from build123d import *

# Parameters (mm, degrees)
SKETCH_1_W          = 11
SKETCH_1_H          = 36
EXTRUDE_1_DEPTH     = 18
SKETCH_2_R          = 7.5
EXTRUDE_2_DEPTH     = 20
FILLET_3_R          = 4
SKETCH_3_R          = 1.5
CUT_EXTRUDE_1_DEPTH = 45.944410108


with BuildPart() as part:
    # 草图1 → 凸台-拉伸1 (new, symmetric)
    with BuildSketch(Plane(origin=(0, 0, 0), x_dir=(0, 0, -1), z_dir=(1, 0, 0))):
        Rectangle(SKETCH_1_W, SKETCH_1_H)
    extrude(amount=EXTRUDE_1_DEPTH, both=True)

    # 草图2 → 凸台-拉伸2 (add)
    with BuildSketch(Plane.XY):
        with Locations(Location((0, 0, 0), (0, 0, 180))):
            Circle(SKETCH_2_R)
    extrude(amount=EXTRUDE_2_DEPTH)

    # 圆角3
    fillet_3_edges = [part.edges().sort_by_distance(p)[0] for p in [
        (7.5, 0, 20),
    ]]
    fillet(fillet_3_edges, radius=FILLET_3_R)

    # 草图3 → 切除-拉伸1 (cut, through all)
    with BuildSketch(Plane.ZY.offset(18)):
        Circle(SKETCH_3_R)
    extrude(amount=-CUT_EXTRUDE_1_DEPTH, mode=Mode.SUBTRACT)


solid = part.part
Model file for the job. Use its own axes, mm. Give positions to 0.01 mm unless a question says otherwise; leave off trailing zeros. Write each loop counter-clockwise with the first axis right and the second up, starting at its lowest first coordinate (ties: lowest second). Pieces come first, ordered by that corner, then holes. Notation, with made-up numbers: (69.5, 68.5) -> (106.5, 68.5) arc R11 ccw to (106.5, 82.5) -> close; hole circle Ø7 at (23, -34). An arc over 180 degrees is marked (long way). Write item = value, one per line.
(1) Slice it at D-D, the plane y = -8. Give the cut face in (x, z).
Determined:
outline = (-18, -5.5) -> (18, -5.5) -> (18, 5.5) -> (-18, 5.5) -> close
(2) Probe line 1 along Y through (x, z) = (1.5, 0); line 2 along Z through (x, y) = (11.5, -4.5); line 3 along Y through (x, z) = (0.5, 12.5). List the from-to ranges inside material, lowest first.
Determined:
line_1 = -18 to -1.5, 1.5 to 18
line_2 = -5.5 to 5.5
line_3 = -7.48 to 7.48
(3) Flat gauge pins, fed straight in: P1, Ø2, axis at x = 10, z = 14, coming from the +Y side; P2, Ø1.5, axis at x = -7.5, z = 13.5, coming from the -Y side; P3, Ø8, axis at x = 3, z = 11.5, coming from the -Y side; P4, Ø1, axis at x = 11, y = 6, coming from the +Z side. Where does each tip first touch, or does it go through?
Determined:
P1 = through
P2 = -3.27
P3 = -7.5
P4 = 5.5
(4) Mould opens along Z. For faces 1 (the face through (0, -8, 5.5)), 2 (the face through (-4.032, -6.324, 10.676)), 3 (the face through (-0.25, 0.07, -1.5)) say: released by +Z, released by -Z, zero draft, split by the parting line, or undercut.
Determined:
face_1 = released by +Z
face_2 = zero draft
face_3 = undercut
(5) Slice it at C-C, the plane z = 10.75. Give the cut face in (x, y), then the cut area to 3 significant figures.
Determined:
outline = circle Ø15 at (0, 0)
area = 177 mm2
(6) Slice it at A-A, the plane z = 0.5. Give the cut face in (x, y), then the cut area to 3 significant figures.
Determined:
outline = (-18, -18) -> (18, -18) -> (18, -1.41) -> (-18, -1.41) -> close; (-18, 1.41) -> (18, 1.41) -> (18, 18) -> (-18, 18) -> close
area = 1,190 mm2
(7) Slice it at B-B, the plane x = -9.5. Give the cut face in (y, z).
Determined:
outline = (-18, -5.5) -> (18, -5.5) -> (18, 5.5) -> (-18, 5.5) -> close; hole circle Ø3 at (0, 0)
